Can you work these out from the drawing? Everything is in mm from the part's minimum corner. A direction names the side the tool comes from. Coordinates: 2 decimals unless noted, no trailing zeros. Order: outer loops, then holes, each group sorted by start corner. A loop starts at its lowest first (then second) coordinate and runs counter-clockwise, first axis right, second up. Notation, with made-up numbers: (-5, -20) -> (49, -20) arc R9 ccw to (49, -6) -> close; hole circle Ø3 at (58, 28). An arc over 180 degrees is marked (long way). Put each result on its own line as item: value. Start each with the question number.
Q1. If we section it at B-B (z = 27.5): Please give me the cut outline in (x, y) (1 decimal).
Q2. For the marked faces 4 and 5, which set-ups out of +Z, -Z, +X, -X, +Y, -Y let a thin tool reach every point of the face, with its end or its side?
Q3. Please list where these lines run through material, in increasing order: line 1 along X through (y, z) = (6, 26.5) (1 decimal); line 2 along Z through (x, y) = (20, 4.75) (1 decimal); line 3 along X through (y, z) = (0.5, 17) (1 decimal).
Q4. We'd pull the mould along Z, two halves only. Please class the marked faces 1, 2 and 3: +Z half, -Z half, draft (parallel to the pull), parting line (faces both ways), or undercut.
Q5. If we section it at C-C (y = 4.5): Please give me the cut outline in (x, z), and give its area (3 significant figures).
Q6. If we section it at A-A (z = 21): Please give me the cut outline in (x, y).
Q7. Will these pins go through, and if not, where does the flat tip stop? pin 1 (2 mm diameter, centred on x = 17, y = 2, fed in from -Z) (1 decimal); pin 2 (1.8 mm diameter, centred on x = 20, z = 6.5, fed in from +Y); pin 3 (3 mm diameter, centred on y = 3.5, z = 18, fed in from +X).
Q8. If we section it at D-D (z = 6): Please give me the cut outline in (x, y), and give its area (3 significant figures).
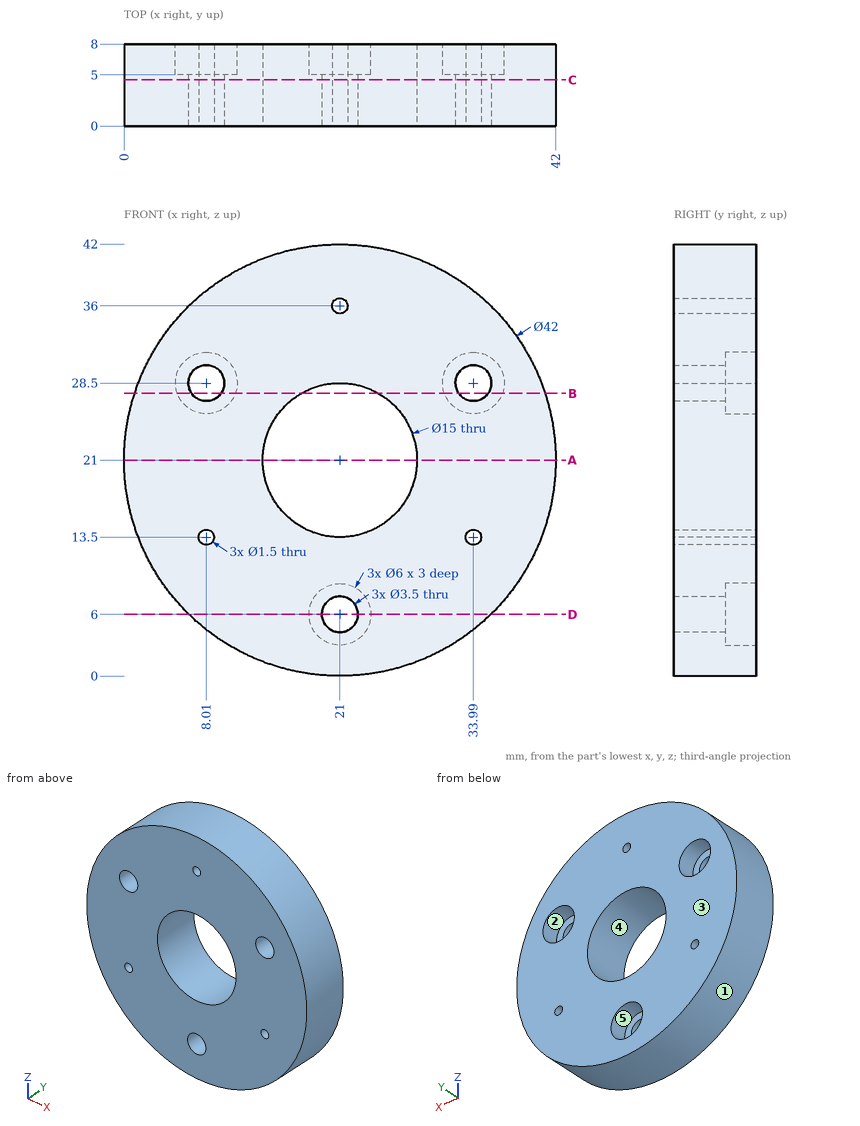
The answers:
1. outline: (1, 0) -> (6.6, 0) -> (6.6, 5) -> (5.2, 5) -> (5.2, 8) -> (1, 8) -> close; (9.4, 0) -> (17.3, 0) -> (17.3, 8) -> (10.8, 8) -> (10.8, 5) -> (9.4, 5) -> close; (24.7, 0) -> (32.6, 0) -> (32.6, 5) -> (31.2, 5) -> (31.2, 8) -> (24.7, 8) -> close; (35.4, 0) -> (41, 0) -> (41, 8) -> (36.8, 8) -> (36.8, 5) -> (35.4, 5) -> close
2. face 4: +Y, -Y
2. face 5: +Y
3. line 1: 0.7 to 5.8, 10.2 to 15.9, 26.1 to 31.8, 36.2 to 41.3
3. line 2: 0 to 4.6, 7.4 to 13.6, 28.4 to 42
3. line 3: 0.4 to 14.7, 27.3 to 41.6
4. face 1: parting line
4. face 2: undercut
4. face 3: draft
5. outline: circle Ø42 at (21, 21); hole circle Ø3.5 at (8.01, 28.5); hole circle Ø1.5 at (8.01, 13.5); hole circle Ø15 at (21, 21); hole circle Ø3.5 at (21, 6); hole circle Ø1.5 at (21, 36); hole circle Ø3.5 at (33.99, 28.5); hole circle Ø1.5 at (33.99, 13.5)
5. area: 1,170 mm^2
6. outline: (0, 0) -> (13.5, 0) -> (13.5, 8) -> (0, 8) -> close; (28.5, 0) -> (42, 0) -> (42, 8) -> (28.5, 8) -> close
7. pin 1: z = 0.2
7. pin 2: y = 5
7. pin 3: x = 41.95
8. outline: (6.3, 0) -> (19.25, 0) -> (19.25, 5) -> (18, 5) -> (18, 8) -> (6.3, 8) -> close; (22.75, 0) -> (35.7, 0) -> (35.7, 8) -> (24, 8) -> (24, 5) -> (22.75, 5) -> close
8. area: 200 mm^2
